from build123d import *

# Parameters (mm, degrees)
SKETCH5_R           = 35
SKETCH5_R_2         = 10
BOSS_EXTRUDE2_DEPTH = 80
SKETCH6_W           = 60
SKETCH6_H           = 25.98
CUT_EXTRUDE3_DEPTH  = 10
SKETCH7_W           = 40
SKETCH7_H           = 36.06
CUT_EXTRUDE4_DEPTH  = 10


with BuildPart() as part:
    # Sketch5 → Boss-Extrude2 (new body)
    with BuildSketch(Plane(origin=(0, 0, 0), x_dir=(0, 0, -1), z_dir=(1, 0, 0))):
        Circle(SKETCH5_R)
        Circle(SKETCH5_R_2, mode=Mode.SUBTRACT)
    extrude(amount=-BOSS_EXTRUDE2_DEPTH)

    # Sketch6 → Cut-Extrude3 (cut)
    with BuildSketch(Plane(origin=(0, 32.5, 0), x_dir=(1, 0, 0), z_dir=(0, 1, 0))):
        with Locations((-40, 0)):
            Rectangle(SKETCH6_W, SKETCH6_H)
    extrude(amount=CUT_EXTRUDE3_DEPTH, mode=Mode.SUBTRACT)

    # Sketch7 → Cut-Extrude4 (cut)
    with BuildSketch(Plane.XY.offset(30)):
        with Locations((-40, 0)):
            Rectangle(SKETCH7_W, SKETCH7_H)
    extrude(amount=CUT_EXTRUDE4_DEPTH, mode=Mode.SUBTRACT)


solid = part.part
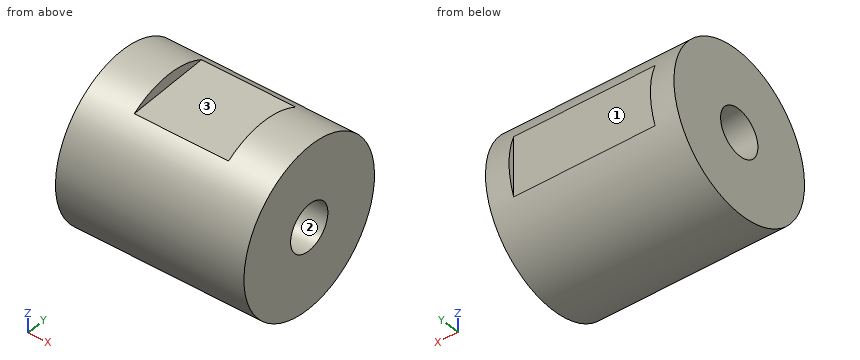
Input: part model. Units: mm. Frame: model coordinates. Face numbers are marked on the shaded views. Give positions to 0.01 mm unless a question says otherwise; leave off trailing zeros. Loops run counter-clockwise (first coordinate to the right, second up) from the corner with the lowest first, then second, coordinate; pieces in that order, holes last. Notation, with made-up numbers: M 71,27 L 90,27 A23 ccw 90,40 Z; hole C 18.5,-16 d2. An arc over 180 degrees is marked long. Use one line per item in the form item = value.
1. Pull-direction query (Y, two-part tool) for the marked faces 1, 2 and 3; classes: released by +Y, released by -Y, zero draft, split by the parting line, or undercut.
Numbers:
face_1 = released by +Y
face_2 = undercut
face_3 = zero draft
2. Section query B-B, the plane y = 0. Return the cut outline in (x, z).
Numbers:
outline = M -80,-35 L 0,-35 L 0,-10 L -80,-10 Z; M -80,10 L 0,10 L 0,35 L -20,35 L -20,30 L -60,30 L -60,35 L -80,35 Z
3. First-contact query: pin 1 (13 mm diameter, centred on x = -45.5, z = 2, fed in from +Y); pin 2 (4 mm diameter, centred on x = -57.5, z = -11.5, fed in from -Y); pin 3 (12 mm diameter, centred on x = -45.5, y = -11.5, fed in from -Z). Flat tips, straight axial feed; report the tip coordinate or a pass-through.
Numbers:
pin_1 = 32.5
pin_2 = -33.69
pin_3 = -34.57
4. Section query A-A, the plane z = 0. Return the cut outline in (x, y), and give its area (3 significant figures).
Numbers:
outline = M -80,-35 L 0,-35 L 0,-10 L -80,-10 Z; M -80,10 L 0,10 L 0,35 L -10,35 L -10,32.5 L -70,32.5 L -70,35 L -80,35 Z
area = 3,850 mm²
5. Line query: L1, parallel to Y at x = -31.5, z = 0; L2, parallel to Y at x = -51, z = 2; L3, parallel to Y at x = -64, z = -30. Output: solid intervals per line, ascending.
Numbers:
L1 = -35 to -10, 10 to 32.5
L2 = -34.94 to -9.8, 9.8 to 32.5
L3 = -18.03 to 18.03
6. Section query D-D, the plane y = -15.5. Return the cut outline in (x, z), and give its area (3 significant figures).
Numbers:
outline = M -80,-31.38 L 0,-31.38 L 0,31.38 L -20,31.38 L -20,30 L -60,30 L -60,31.38 L -80,31.38 Z
area = 4,970 mm²
